Work out the finished part from the listing and answer in its coordinate system (mm). A direction names the side the tool comes from. Round coordinates to 2 decimals unless told otherwise and drop trailing zeros. Loops run counter-clockwise (first coordinate to the right, second up) from the corner with the lowest first, then second, coordinate; pieces in that order, holes last.
```python
from build123d import *

# Parameters (mm, degrees)
F0_W     = 150
F0_H     = 90
F1_DEPTH = 72
F2_W     = 70
F2_H     = 12
F3_DEPTH = 25
F4_W     = 150
F4_H     = 20
F5_DEPTH = 60


with BuildPart() as f1:
    # F0 (on Top) → F1 (new body)
    with BuildSketch(Plane.XY):
        Rectangle(F0_W, F0_H)
    extrude(amount=F1_DEPTH)

    # F2 (on face) → F3 (cut)
    with BuildSketch(Plane.XY.offset(72)):
        with Locations((-40, -31)):
            Rectangle(F2_W, F2_H)
        with Locations((40, -31)):
            Rectangle(F2_W, F2_H)
    extrude(amount=-F3_DEPTH, mode=Mode.SUBTRACT)

    # F4 (on face) → F5 (cut)
    with BuildSketch(Plane.XY.offset(72)):
        with Locations((0, 25)):
            Rectangle(F4_W, F4_H)
        with Locations((0, -5)):
            Rectangle(F4_W, F4_H)
    extrude(amount=-F5_DEPTH, mode=Mode.SUBTRACT)


solid = f1.part
```
1. Find section D-D (z = 18.5). Write down the section's boundary in (x, y), then the cut area to 3 significant figures.
Answer key:
outline: (-75, -45) - (75, -45) - (75, -15) - (-75, -15) - close; (-75, 5) - (75, 5) - (75, 15) - (-75, 15) - close; (-75, 35) - (75, 35) - (75, 45) - (-75, 45) - close
area: 7,500 mm2
2. Find section C-C (y = -32.5). Write down the section's boundary in (x, z).
Answer key:
outline: (-75, 0) - (75, 0) - (75, 47) - (5, 47) - (5, 72) - (-5, 72) - (-5, 47) - (-75, 47) - close
3. Which of the six approach directions +Z, -Z, +X, -X, +Y, -Y give full straight-line access (tool end or side, diameter ignored) to faces 1 (the face through (-1, 35, 42)), 2 (the face through (-40, -37, 60)), 3 (the face through (40, -25, 60))?
Answer key:
face 1: +Z, +X, -X
face 2: +Z, -X
face 3: +Z, +X
4. Find section A-A (z = 66). Write down the section's boundary in (x, y), then the cut area to 3 significant figures.
Answer key:
outline: (-75, -45) - (75, -45) - (75, -37) - (5, -37) - (5, -25) - (75, -25) - (75, -15) - (-75, -15) - (-75, -25) - (-5, -25) - (-5, -37) - (-75, -37) - close; (-75, 5) - (75, 5) - (75, 15) - (-75, 15) - close; (-75, 35) - (75, 35) - (75, 45) - (-75, 45) - close
area: 5,820 mm2
5. Given pin 1 (6 mm diameter, centred on x = 29, y = -7.5, fed in from +Z); pin 2 (3.5 mm diameter, centred on x = -23.5, y = -32.5, fed in from +Z); pin 3 (6 mm diameter, centred on y = -28.5, z = 65, fed in from +X), each flat-ended and moving along its own axis, determine where each tip first touches the part or whether it passes through.
Answer key:
pin 1: stops at z = 12
pin 2: stops at z = 47
pin 3: stops at x = 5
6. Find section B-B (x = -58.5). Write down the section's boundary in (y, z), then the cut area to 3 significant figures.
Answer key:
outline: (-45, 0) - (45, 0) - (45, 72) - (35, 72) - (35, 12) - (15, 12) - (15, 72) - (5, 72) - (5, 12) - (-15, 12) - (-15, 72) - (-25, 72) - (-25, 47) - (-37, 47) - (-37, 72) - (-45, 72) - close
area: 3,780 mm2
7. Consider probe 1 along Y at (x, z) = (42, 23.5); probe 2 along Y at (x, z) = (-56, 56); probe 3 along Z at (x, y) = (41, -8). Determine where each line is inside the solid, lowest interval first.
Answer key:
probe 1: y = -45 to -15, 5 to 15, 35 to 45
probe 2: y = -45 to -37, -25 to -15, 5 to 15, 35 to 45
probe 3: z = 0 to 12
8. Determine the mould class of faces 4 (the face through (-1, 5, 42)), 5 (the face through (75, 9, 27)), 6 (the face through (-1, -45, 35)) for opening direction Y: +Y half, -Y half, draft (parallel to the pull), parting line (faces both ways), or undercut.
Answer key:
face 4: undercut
face 5: draft
face 6: -Y half
